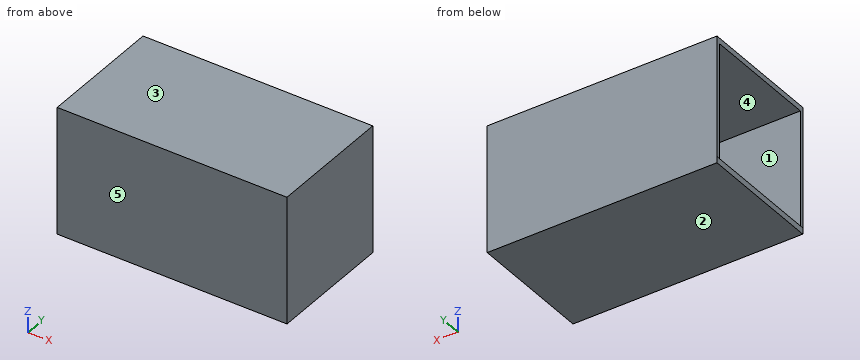
```python
from build123d import *

# Parameters (mm, degrees)
SKETCH_1_W          = 82
SKETCH_1_H          = 30
EXTRUDE_1_DEPTH     = 1.5
SKETCH_2_W          = 1.997612732
SKETCH_2_H          = 25.79850023
EXTRUDE_3_DEPTH     = 3.5
SKETCH_4_W          = 1.75
SKETCH_4_H          = 25.79850023
EXTRUDE_4_DEPTH     = 26
SKETCH_5_W          = 55.064096776
SKETCH_5_H          = 30
EXTRUDE_5_DEPTH     = 29
SKETCH_6_W          = 26.352675357
SKETCH_6_H          = 28.194959652
CUT_EXTRUDE_1_DEPTH = 53
SKETCH_8_W          = 53
SKETCH_8_H          = 28.194959652
CUT_EXTRUDE_2_DEPTH = 1.32
CUT_EXTRUDE_5_DEPTH = 26.94
CUT_EXTRUDE_6_DEPTH = 26.94


with BuildPart() as part:
    # 草圖1 → 填料-伸長1 (new body)
    with BuildSketch(Plane.XY):
        Rectangle(SKETCH_1_W, SKETCH_1_H)
    extrude(amount=EXTRUDE_1_DEPTH)

    # 草圖2 → 填料-伸長3 (add)
    with BuildSketch(Plane(origin=(0, 0, 0), x_dir=(-1, 0, 0), z_dir=(0, 0, -1))):
        with Locations((40.001193634, 0)):
            Rectangle(SKETCH_2_W, SKETCH_2_H)
    extrude(amount=EXTRUDE_3_DEPTH)

    # 草圖4 → 填料-伸長4 (add)
    with BuildSketch(Plane(origin=(-39.002387268, 0, 0), x_dir=(0, 0, -1), z_dir=(1, 0, 0))):
        with Locations((2.625, 0)):
            Rectangle(SKETCH_4_W, SKETCH_4_H)
    extrude(amount=EXTRUDE_4_DEPTH)

    # 草圖5 → 填料-伸長5 (add)
    with BuildSketch(Plane.XY.offset(1.5)):
        with Locations((13.467951612, 0)):
            Rectangle(SKETCH_5_W, SKETCH_5_H)
    extrude(amount=EXTRUDE_5_DEPTH)

    # 草圖6 → 除料-伸長1 (cut)
    with BuildSketch(Plane.ZY.offset(14.064096776)):
        with Locations((15.993727328, -0.060074488)):
            Rectangle(SKETCH_6_W, SKETCH_6_H)
    extrude(amount=-CUT_EXTRUDE_1_DEPTH, mode=Mode.SUBTRACT)

    # 草圖8 → 除料-伸長2 (cut)
    with BuildSketch(Plane.XY.offset(2.817389649)):
        with Locations((12.435903224, -0.060074488)):
            Rectangle(SKETCH_8_W, SKETCH_8_H)
    extrude(amount=-CUT_EXTRUDE_2_DEPTH, mode=Mode.SUBTRACT)

    # 草圖10 → 除料-伸長5 (cut)
    with BuildSketch(Plane.ZY.offset(41)):
        Polygon((1.5, 15), (1.5, -16.079937927), (-4.357490946, -16.079937927), (-4.357490946, 16.240136561), (1.5, 16.240136561), align=None)
    extrude(amount=-CUT_EXTRUDE_5_DEPTH, mode=Mode.SUBTRACT)


with BuildPart() as cut_extrude_5_piece_1:
    # of the separate pieces the step leaves, piece 1, a body of its own (cut_extrude_5_pieces)
    add(part.part.solids().sort_by_distance((-14.06, 15, 0))[0])


with BuildPart() as cut_extrude_5_piece_2:
    # of the separate pieces the step leaves, piece 2, a body of its own (cut_extrude_5_pieces)
    add(part.part.solids().sort_by_distance((-14.06, 12.899250115, -1.75))[0])

    # 草圖11 → 除料-伸長6 (cut)
    with BuildSketch(Plane.ZY.offset(14.06)):
        Polygon((-1.75, 12.899250115), (-3.5, 12.899250115), (-4.749423893, -13.676958411), (-1.265103595, -13.676958411), (-1.265103595, 12.899250115), align=None)
    extrude(amount=-CUT_EXTRUDE_6_DEPTH, mode=Mode.SUBTRACT)


solid = cut_extrude_5_piece_1.part
```
Geometry check sheet. Reference: the model listing, model coordinates, mm. Face numbers are marked on the shaded views. A direction names the side the tool comes from. Round coordinates to 2 decimals unless told otherwise and drop trailing zeros. Write each loop counter-clockwise with the first axis right and the second up, starting at its lowest first coordinate (ties: lowest second). Pieces come first, ordered by that corner, then holes. Notation, with made-up numbers: (36, 89.5) -> (41, 89.5) arc R21 cw to (41, 101.5) -> close; hole circle Ø1 at (31.5, 52). An arc over 180 degrees is marked (long way). Put each result on its own line as item: value.
1) Release check for a two-part mould opening along Z. For the marked faces 3, 4 and 5 record: pulls with the +Z half, pulls with the -Z half, needs draft (parallel to the pull), parting line crosses it, or undercut.
Recorded:
face 3: pulls with the +Z half
face 4: undercut
face 5: needs draft
2) Thickness scan on probe 1 along Y at (x, z) = (27.5, 17.5); probe 2 along Z at (x, y) = (4.5, -9.5); probe 3 along X at (y, z) = (13.25, 20.5). Record the ranges inside material, lowest first. Write a range as from..to.
Recorded:
probe 1: y = -15..-14.16, 14.04..15
probe 2: z = 0..1.5, 29.17..30.5
probe 3: x = 38.94..41
3) Access from +Z, -Z, +X, -X, +Y, -Y to the whole of each face (thin tool, end or side, straight path). Record for the marked faces 1 and 2.
Recorded:
face 1: -X
face 2: -Z, +X, -X, +Y, -Y
4) Cross-section at B-B, the plane z = 11. Enter the section's corners in (x, y).
Recorded:
outline: (-14.06, -15) -> (41, -15) -> (41, 15) -> (-14.06, 15) -> (-14.06, 14.04) -> (38.94, 14.04) -> (38.94, -14.16) -> (-14.06, -14.16) -> close
5) Cross-section at C-C, the plane y = -0.75. Enter the section's corners in (x, z).
Recorded:
outline: (-14.06, 0) -> (41, 0) -> (41, 30.5) -> (-14.06, 30.5) -> (-14.06, 29.17) -> (38.94, 29.17) -> (38.94, 1.5) -> (-14.06, 1.5) -> close
6) Depth check by flat-ended pin: P1, Ø14, axis at y = 1.5, z = 16.5, coming from the -X side; P2, Ø1.6, axis at y = 1, z = 1, coming from the -X side. Enter the tip coordinate at first touch or a pass-through.
Recorded:
P1: stops at x = 38.94
P2: stops at x = -14.06
7) Cross-section at A-A, the plane x = 7.5. Enter the section's corners in (y, z), plus the area to 3 significant figures.
Recorded:
outline: (-15, 0) -> (15, 0) -> (15, 30.5) -> (-15, 30.5) -> close; hole (-14.16, 1.5) -> (14.04, 1.5) -> (14.04, 29.17) -> (-14.16, 29.17) -> close
area: 135 mm2
